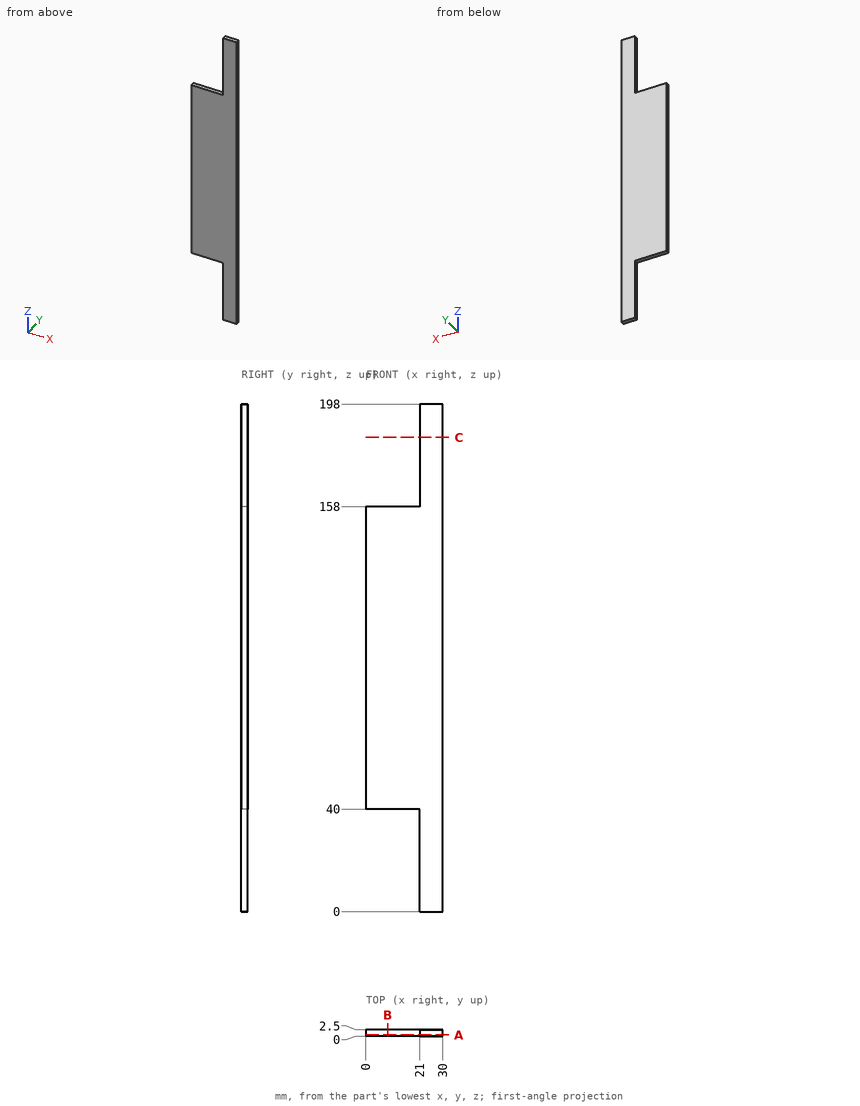
Drawing for the job (mm, zero at the part's lowest x, y, z). Round coordinates to 2 decimals unless told otherwise and drop trailing zeros. Loops run counter-clockwise (first coordinate to the right, second up) from the corner with the lowest first, then second, coordinate; pieces in that order, holes last. Notation, with made-up numbers: (-26.75, 60) -> (15.25, 60) arc R24 ccw to (15.25, 76) -> close; hole circle Ø5 at (11, 64). An arc over 180 degrees is marked (long way). Answer in a Markdown table with one row per item.
Item 1: Pin check, flat tips, straight feed: pin 1 (1.5 mm diameter, centred on x = 20, y = 1.5, fed in from -Z); pin 2 (3 mm diameter, centred on x = 18.5, z = 128.5, fed in from -Y). Stop position of each tip, or through.
Answers below:
| item | result |
|---|---|
| pin 1 | stops at z = 40 |
| pin 2 | stops at y = 0 |
Item 2: Saw through at B-B (x = 8.5). Write the cut outline in (y, z), and give its area (3 significant figures).
Answers below:
| item | result |
|---|---|
| outline | (0, 40) -> (2.5, 40) -> (2.5, 158) -> (0, 158) -> close |
| area | 295 mm² |
Item 3: Drill centre lines: L1, parallel to Z at x = 3.5, y = 2.4; L2, parallel to X at y = 1.75, z = 27. Where is each one in solid material? Low to high. Write a range as [from, to].
Answers below:
| item | result |
|---|---|
| L1 | z = [40, 158] |
| L2 | x = [21, 30] |
Item 4: Saw through at C-C (z = 185). Write the cut outline in (x, y).
Answers below:
| item | result |
|---|---|
| outline | (21, 0) -> (30, 0) -> (30, 2.5) -> (21, 2.5) -> close |
Item 5: Saw through at A-A (y = 0.45). Write the cut outline in (x, z), and give its area (3 significant figures).
Answers below:
| item | result |
|---|---|
| outline | (0, 40) -> (21, 40) -> (21, 0) -> (30, 0) -> (30, 198) -> (21, 198) -> (21, 158) -> (0, 158) -> close |
| area | 4,260 mm² |
